Can you work these out from the model? Positions are in its coordinate system, mm. Face numbers are marked on the shaded views. Round coordinates to 2 decimals unless told otherwise and drop trailing zeros. Loops run counter-clockwise (first coordinate to the right, second up) from the corner with the lowest first, then second, coordinate; pieces in that order, holes last. Notation, with made-up numbers: (79, 47) -> (125, 47) arc R16 cw to (125, 76) -> close; hole circle Ø3 at (-25, 68). An arc over 180 degrees is marked (long way). Use a Markdown table: item, result.
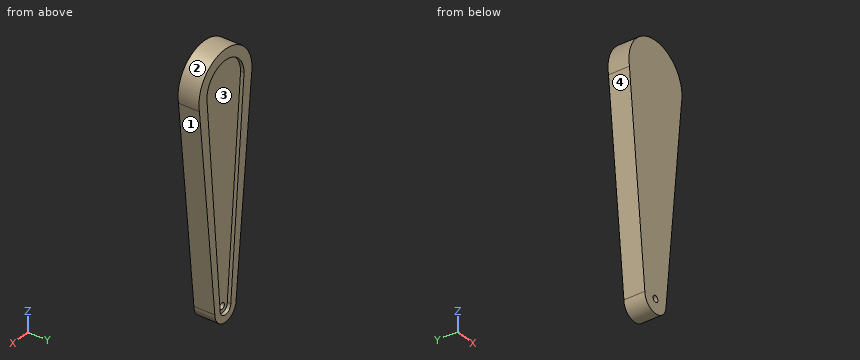
Autodesk Inventor part; units mm, degrees
ref_plane "YZ Plane" through (0, 0, 0) normal (1, 0, 0) x (0, 1, 0)
ref_plane "XZ Plane" through (0, 0, 0) normal (0, 1, 0) x (-1, 0, 0)
ref_plane "XY Plane" through (0, 0, 0) normal (0, 0, 1) x (1, 0, 0)
sketch "Sketch1" plane through (0, 0, 0) normal (0, 1, 0) x (-1, 0, 0)
  circle A0 centre (0, 0) radius 25
  line L0 (0, 0) -> (0, -150)
  circle A1 centre (0, -150) radius 10
  line L1 (0, 0) -> (25, 0)
  line L2 (0, -150) -> (10, -150)
  line L3 (0, -150) -> (-10, -150)
  line L4 (0, 0) -> (-25, 0)
  line L5 (25, 0) -> (10, -150)
  line L6 (-25, 0) -> (-10, -150)
  dimension "d0" = 50
  dimension "d1" = 150
  dimension "d2" = 20
extrude "Extrusion1" add sketch "Sketch1" along normal blind 15
sketch "Sketch2" plane through (0, 15, 0) normal (0, 1, 0) x (1, 0, 0)
  circle A0 centre (0, 0) radius 17.5
  arc A1 (10, 150) -> (-10, 150) centre (0, 150) ccw
  circle A2 centre (0, 150) radius 5
  line L0 (0, 0) -> (-17.5, 0)
  line L1 (0, 0) -> (17.5, 0)
  line L2 (0, 150) -> (-5, 150)
  line L3 (0, 150) -> (5, 150)
  line L4 (-17.5, 0) -> (-5, 150)
  line L5 (5, 150) -> (17.5, 0)
  dimension "d5" = 35
  dimension "d6" = 10
extrude "Extrusion2" cut sketch "Sketch2" against normal blind 2.5 contours L0 L1 A0 | L4 A0 L5 L1 L0 | L4 A2 L5 A0 | L2 L3 A2 | A2 L3 L2
sketch "Sketch3" plane through (0, 12.5, 0) normal (0, 1, 0) x (1, 0, 0)
  arc A0 (5, 150) -> (-5, 150) centre (0, 150) ccw
  circle A1 centre (0, 150) radius 2.25
  point P0 (0, 0)
  dimension "d9" = 4.5
extrude "Extrusion3" cut sketch "Sketch3" against normal blind 12.5
properties part number "Delta_Arm"
1. I want a section at A-A (x = 0). Please give me the cut outline in (y, z).
Answer sheet:
| item | result |
|---|---|
| outline | (0, -160) -> (15, -160) -> (15, -155) -> (12.5, -155) -> (12.5, -152.25) -> (0, -152.25) -> close; (0, -147.75) -> (12.5, -147.75) -> (12.5, 17.5) -> (15, 17.5) -> (15, 25) -> (0, 25) -> close |
2. I want a section at C-C (z = -87). Please give me the cut outline in (x, y).
Answer sheet:
| item | result |
|---|---|
| outline | (-16.3, 0) -> (16.3, 0) -> (16.3, 15) -> (10.25, 15) -> (10.25, 12.5) -> (-10.25, 12.5) -> (-10.25, 15) -> (-16.3, 15) -> close |
3. Will these pins go through, and if not, where does the flat tip stop? pin 1 Ø6 at (x, z) = (-5.5, -13.5) entering from +Y; pin 2 Ø2 at (y, z) = (13.5, -63) entering from -X; pin 3 Ø6 at (y, z) = (12, -134.5) entering from -X.
Answer sheet:
| item | result |
|---|---|
| pin 1 | stops at y = 12.5 |
| pin 2 | stops at x = -18.8 |
| pin 3 | stops at x = -11.85 |
4. I want a section at D-D (x = -15.5). Please give me the cut outline in (y, z).
Answer sheet:
| item | result |
|---|---|
| outline | (0, -95) -> (15, -95) -> (15, -24) -> (12.5, -24) -> (12.5, 8.12) -> (15, 8.12) -> (15, 19.62) -> (0, 19.62) -> close |
5. I need wall thicknesses on line 1 (Z direction, x = 0, y = 10.25); line 2 (X direction, y = 7.5, z = -150); line 3 (Y direction, x = -12, z = -39). Which ranges of each line are inside material? Lowest first, please.
Answer sheet:
| item | result |
|---|---|
| line 1 | z = -160 to -152.25, -147.75 to 25 |
| line 2 | x = -10 to -2.25, 2.25 to 10 |
| line 3 | y = 0 to 12.5 |
6. If we mould it in two halves opening along X, with no side actions, what happens to the marked faces 1, 2, 3 and 4? For each: +X half, -X half, draft (parallel to the pull), parting line (faces both ways), or undercut.
Answer sheet:
| item | result |
|---|---|
| face 1 | +X half |
| face 2 | parting line |
| face 3 | undercut |
| face 4 | -X half |
7. I want a section at B-B (y = 4.25). Please give me the cut outline in (x, z), plus the area to 3 significant figures.
Answer sheet:
| item | result |
|---|---|
| outline | (-24.5, -4.95) -> (-10, -150) arc R10 ccw to (10, -150) -> (24.5, -4.95) arc R25 ccw (long way) to start; hole circle Ø4.5 at (0, -150) |
| area | 6,370 mm² |
